Design review of the part built by this model. Coordinates are the model's own, in mm. Round coordinates to 2 decimals unless told otherwise and drop trailing zeros. Order: outer loops, then holes, each group sorted by start corner. A loop starts at its lowest first (then second) coordinate and runs counter-clockwise, first axis right, second up. Notation, with made-up numbers: M 54.25,47.5 L 68.25,47.5 A30 ccw 68.25,76.5 Z; hole C 83.25,23.25 d7. An arc over 180 degrees is marked long. Write item = value, one per line. Start each with the question number.
```python
from build123d import *

# Parameters (mm, degrees)
IZIM2_R               = 2.425
BO_ALTMA1_T           = -1
IZIM3_R               = 2.25
KES_EKSTR_ZYON1_DEPTH = 109


with BuildPart() as part:
    # Süpür1: sweep along a path in Çizim1
    with BuildLine(Plane(origin=(0, 0, 0), x_dir=(0, 0, -1), z_dir=(1, 0, 0))) as s_p_r1_path:
        Line((0, 350), (0, 430))
        ThreePointArc((0, 430), (20.502525317, 479.497474683), (70, 500))
        Line((70, 500), (100, 500))
    # Çizim2 → Süpür1 (sweep)
    with BuildSketch(Plane(origin=(0, 500, -100), x_dir=(-1, 0, 0), z_dir=(0, 0, -1))):
        Circle(IZIM2_R)
    sweep(path=s_p_r1_path.line)

    # İç Boşaltma1
    bo_altma1_openings = [part.faces().sort_by_distance(p)[0] for p in [
        (0, 500, -100),
    ]]
    offset(amount=BO_ALTMA1_T, openings=bo_altma1_openings, kind=Kind.INTERSECTION)

    # Çizim3 → Kes-Ekstrüzyon1 (cut)
    with BuildSketch(Plane.XZ.offset(-350)):
        with Locations(Location((0, 0, 0), (0, 0, 270))):
            Circle(IZIM3_R)
    extrude(amount=-KES_EKSTR_ZYON1_DEPTH, mode=Mode.SUBTRACT)


solid = part.part
```
(1) Consider section C-C, the plane z = -81. Write out the cut boundary in (x, y) (3 decimals), then the cut area to 3 significant figures.
(2) Consider section B-B, the plane y = 421. Write out the cut boundary in (x, z) (3 decimals).
(3) For line 1 along Y through (x, z) = (0, -92) (3 decimals); line 2 along X through (y, z) = (500, -78) (3 decimals); line 3 along Z through (x, y) = (0, 389.5) (3 decimals), list the stretches that pass through material, from the lowest coordinate up. Write a range as [from, to].
(4) Draft analysis for pull direction Z (two halves, no side actions). For faces 1 (the face through (-2, 500, -100)), 2 (the face through (0.676, 390.327, -2.146)), 3 (the face through (-2.313, 390.56, 0.728)), 4 (the face through (0.31, 498.61, -85.21)), state which applies: pulls with the +Z half, pulls with the -Z half, needs draft (parallel to the pull), parting line crosses it, or undercut.
(5) Consider section A-A, the plane x = 0. Write out the cut boundary in (y, z) (3 decimals).
Completed:
q1.outline = C 0,500 d4.85; hole C 0,500 d2.85
q1.area = 12.1 mm2
q2.outline = C 0,0 d4.85; hole C 0,0 d4.5
q3.line_1 = [497.575, 498.575], [501.425, 502.425]
q3.line_2 = [-2.425, -1.425], [1.425, 2.425]
q3.line_3 = [-2.425, -2.25], [2.25, 2.425]
q4.face_1 = pulls with the -Z half
q4.face_2 = undercut
q4.face_3 = parting line crosses it
q4.face_4 = needs draft
q5.outline = M 350,-2.425 L 430,-2.425 A67.575 cw 497.575,-70 L 497.575,-100 L 498.575,-100 L 498.575,-70 A68.575 ccw 440.605,-2.25 L 350,-2.25 Z; M 350,2.25 L 435.032,2.25 A72.425 ccw 430,2.425 L 350,2.425 Z; M 452.616,-2.25 A71.425 cw 501.425,-70 L 501.425,-100 L 502.425,-100 L 502.425,-70 A72.425 ccw 455.599,-2.25 Z
